The listing builds one solid part. Answer for the finished solid, in the listing's coordinates (mm). Round coordinates to 2 decimals unless told otherwise and drop trailing zeros. Order: outer loops, then holes, each group sorted by start corner. A loop starts at its lowest first (then second) coordinate and runs counter-clockwise, first axis right, second up. Notation, with made-up numbers: (-5, 47) -> (34, 47) arc R23 cw to (34, 58) -> close; hole circle Ø2 at (-26, -38). An arc over 180 degrees is marked (long way). Answer in a Markdown table with one row per item. Add a question column.
```python
from build123d import *

# Parameters (mm, degrees)
F0_R     = 10
F0_R_2   = 2.5
F1_DEPTH = 10
F2_SIZE  = 3
F3_R     = 2


with BuildPart() as f1:
    # F0 (on Top) → F1 (new body)
    with BuildSketch(Plane.XY):
        Circle(F0_R)
        Circle(F0_R_2, mode=Mode.SUBTRACT)
    extrude(amount=F1_DEPTH)

    # F2
    f2_edges = [f1.edges().sort_by_distance(p)[0] for p in [
        (-2.5, 0, 10),
    ]]
    chamfer(f2_edges, length=F2_SIZE)

    # F3
    f3_edges = [f1.edges().sort_by_distance(p)[0] for p in [
        (-10, 0, 10),
    ]]
    fillet(f3_edges, radius=F3_R)


solid = f1.part
```
1. The part is cut by section D-D (z = 3.5). Give the vertices of the cut face in (x, y).
2. The mould has two halves that part along X. Classify faces 1 (the cylindrical face through (-2.17, -9.76, 3.94)), 2 (the flat face through (2, -2, 0)), 3 (the cylindrical face through (-0.54, -2.44, 3.45)): released by +X, released by -X, zero draft, split by the parting line, or undercut.
3. Each of these flat-tipped pins is pushed along its axis until it touches: pin 1 (3 mm diameter, centred on y = -7, z = 6.5, fed in from -X); pin 2 (5 mm diameter, centred on y = -6.5, z = 4.5, fed in from -X); pin 3 (8 mm diameter, centred on x = 0, y = 0, fed in from -Z); pin 4 (5 mm diameter, centred on y = -3, z = 4, fed in from -X). Where does it stop, or does it pass through?
4. The part is cut by section C-C (z = 7.75). Give the vertices of the cut face in (x, y).
5. Straight lines are drawn through the part: line 1 along Y through (x, z) = (0, 1.5); line 2 along Y through (x, z) = (6, 4.5); line 3 along Y through (x, z) = (-1.75, 2.25). For each, find the intervals that lie inside material, in ascending order.
6. The part is cut by section A-A (x = 0). Give the vertices of the cut face in (y, z), then the cut area to 3 significant figures.
Report:
| question | item | result |
|---|---|---|
| 1 | outline | circle Ø20 at (0, 0); hole circle Ø5 at (0, 0) |
| 2 | face 1 | split by the parting line |
| 2 | face 2 | zero draft |
| 2 | face 3 | undercut |
| 3 | pin 1 | stops at x = -8.35 |
| 3 | pin 2 | stops at x = -9.17 |
| 3 | pin 3 | stops at z = 0 |
| 3 | pin 4 | stops at x = -9.99 |
| 4 | outline | circle Ø20 at (0, 0); hole circle Ø6.5 at (0, 0) |
| 5 | line 1 | y = -10 to -2.5, 2.5 to 10 |
| 5 | line 2 | y = -8 to 8 |
| 5 | line 3 | y = -9.85 to -1.79, 1.79 to 9.85 |
| 6 | outline | (-10, 0) -> (-2.5, 0) -> (-2.5, 7) -> (-5.5, 10) -> (-8, 10) arc R2 ccw to (-10, 8) -> close; (2.5, 0) -> (10, 0) -> (10, 8) arc R2 ccw to (8, 10) -> (5.5, 10) -> (2.5, 7) -> close |
| 6 | area | 139 mm^2 |
